from build123d import *

# Parameters (mm, degrees)
BOSS_EXTRUDE3_DEPTH = 28
FILLET1_R           = 10
SKETCH8_R           = 9.5
SKETCH8_W           = 8
SKETCH8_H           = 5
CUT_EXTRUDE4_DEPTH  = 5
SKETCH10_R          = 1.75
CUT_EXTRUDE6_DEPTH  = 10
CUT_EXTRUDE9_DEPTH  = 5
SKETCH11_W          = 178.461857567
SKETCH11_H          = 75.855450753
CUT_EXTRUDE7_DEPTH  = 56
SKETCH15_W          = 24.76037583
SKETCH15_H          = 40.698494869
CUT_EXTRUDE10_DEPTH = 39


with BuildPart() as part:
    # Sketch7 → Boss-Extrude3 (new body)
    with BuildSketch(Plane.XY):
        with BuildLine():
            Line((-29.009247715, -3.56026037), (114.990752285, -3.56026037))
            ThreePointArc((114.990752285, -3.56026037), (122.672406567, -0.574706865), (126.321710983, 6.81473963))
            Line((126.321710983, 6.81473963), (124.563663285, 6.81473963))
            ThreePointArc((124.563663285, 6.81473963), (105.365752285, 7.81473963), (124.563663285, 8.81473963))
            Line((124.563663285, 8.81473963), (126.321710983, 8.81473963))
            ThreePointArc((126.321710983, 8.81473963), (125.754505842, 11.49335817), (124.563663285, 13.958842494))
            Line((124.563663285, 13.958842494), (124.563663285, 33.43973963))
            Line((124.563663285, 33.43973963), (96.563663285, 33.43973963))
            Line((96.563663285, 33.43973963), (96.563663285, 1.43973963))
            Line((96.563663285, 1.43973963), (-10.582158714, 1.43973963))
            Line((-10.582158714, 1.43973963), (-10.582158714, 33.43973963))
            Line((-10.582158714, 33.43973963), (-38.582158714, 33.43973963))
            Line((-38.582158714, 33.43973963), (-38.582158714, 13.958842494))
            ThreePointArc((-38.582158714, 13.958842494), (-39.773001272, 11.49335817), (-40.340206412, 8.81473963))
            Line((-40.340206412, 8.81473963), (-38.582158714, 8.81473963))
            ThreePointArc((-38.582158714, 8.81473963), (-19.384247715, 7.81473963), (-38.582158714, 6.81473963))
            Line((-38.582158714, 6.81473963), (-40.340206412, 6.81473963))
            ThreePointArc((-40.340206412, 6.81473963), (-36.690901996, -0.574706865), (-29.009247715, -3.56026037))
        make_face()
    extrude(amount=BOSS_EXTRUDE3_DEPTH)

    # Fillet1
    fillet1_edges = [part.edges().sort_by_distance(p)[0] for p in [
        (-10.582158714, 1.43973963, 14),
        (96.563663285, 1.43973963, 14),
    ]]
    fillet(fillet1_edges, radius=FILLET1_R)

    # Sketch8 → Cut-Extrude4 (cut)
    with BuildSketch(Plane(origin=(0, 1.43973963, 0), x_dir=(1, 0, 0), z_dir=(0, 1, 0))):
        with Locations(Location((63.990752285, -14, 0), (0, 0, 270))):
            Circle(SKETCH8_R)
        with Locations(Location((21.990752285, -14, 0), (0, 0, 270))):
            Circle(SKETCH8_R)
        with Locations((42.990752285, -14)):
            Rectangle(SKETCH8_W, SKETCH8_H)
    extrude(amount=-CUT_EXTRUDE4_DEPTH, mode=Mode.SUBTRACT)

    # Sketch10 → Cut-Extrude6 (cut)
    with BuildSketch(Plane(origin=(0, 33.43973963, 0), x_dir=(1, 0, 0), z_dir=(0, 1, 0))):
        with Locations(Location((110.490752285, -14, 0), (0, 0, 180))):
            Circle(SKETCH10_R)
        with Locations(Location((-24.509247715, -14, 0), (0, 0, 180))):
            Circle(SKETCH10_R)
    extrude(amount=-CUT_EXTRUDE6_DEPTH, mode=Mode.SUBTRACT)

    # Sketch13 → Cut-Extrude9 (cut)
    with BuildSketch(Plane(origin=(0, 33.43973963, 0), x_dir=(1, 0, 0), z_dir=(0, 1, 0))):
        Polygon((108.61436391, -17.25), (112.36714066, -17.25), (114.243529035, -14), (112.36714066, -10.75), (108.61436391, -10.75), (106.737975536, -14), align=None)
        Polygon((-20.756470965, -14), (-22.63285934, -10.75), (-26.38563609, -10.75), (-28.262024464, -14), (-26.38563609, -17.25), (-22.63285934, -17.25), align=None)
    extrude(amount=-CUT_EXTRUDE9_DEPTH, mode=Mode.SUBTRACT)

    # Sketch11 → Cut-Extrude7 (cut)
    with BuildSketch(Plane.XY.offset(28)):
        with Locations((7.260936379, 24.571309344)):
            Rectangle(SKETCH11_W, SKETCH11_H)
    extrude(amount=-CUT_EXTRUDE7_DEPTH, mode=Mode.SUBTRACT)

    # Sketch15 → Cut-Extrude10 (cut)
    with BuildSketch(Plane.ZY.offset(-96.491865162)):
        with Locations((20.2732889, 14.243484204)):
            Rectangle(SKETCH15_W, SKETCH15_H)
    extrude(amount=-CUT_EXTRUDE10_DEPTH, mode=Mode.SUBTRACT)


solid = part.part
The listing builds one solid part. Answer for the finished solid, in the listing's coordinates (mm). A direction names the side the tool comes from. Give positions to 0.01 mm unless a question says otherwise; leave off trailing zeros. Write each loop counter-clockwise with the first axis right and the second up, starting at its lowest first coordinate (ties: lowest second). Pieces come first, ordered by that corner, then holes.
Item 1: Section C-C, the plane z = 4.75 is taken. Write down the section's boundary in (x, y) (3 decimals), plus the area to 3 significant figures.
Item 2: Find the intervals of material crossed by line 1 along X through (y, z) = (20.5, 6.5); line 2 along Y through (x, z) = (112.5, 4); line 3 along X through (y, z) = (1, 6.25), in increasing order.
Item 3: Section B-B, the plane y = 1 is taken. Write down the section's boundary in (x, z), plus the area to 3 significant figures.
Item 4: Which of the six approach directions +Z, -Z, +X, -X, +Y, -Y give full straight-line access (tool end or side, diameter ignored) to faces 4 (the flat face through (106, -3.56, 4)), 5 (the flat face through (125, 8.815, 4)), 6 (the flat face through (96.564, 23, 4))?
Item 5: Determine the mould class of faces 1 (the flat face through (124.564, 24, 4)), 2 (the flat face through (111, 33.44, 4)), 3 (the cylindrical face through (105.374, 7.406, 3.891)) for opening direction X: released by +X, released by -X, zero draft, split by the parting line, or undercut.
Item 6: Section D-D, the plane y = 29.5 is taken. Write down the section's boundary in (x, z), plus the area to 3 significant figures.
Item 7: Flat-ended cylindrical pins translate along their axes: P1, Ø1.4, axis at x = 125.5, z = 2.5, coming from the -Y side; P2, Ø1.5, axis at x = 123, z = 3, coming from the -Y side; P3, Ø2.5, axis at y = 21.5, z = 4.5, coming from the -X side. Find the tip coordinate at first contact, or state that the pin passes through.
Item 8: Section A-A, the plane x = 106 is taken. Write down the section's boundary in (y, z).
Completed:
1. outline: (96.492, -3.56) - (114.991, -3.56) arc R11.375 ccw to (126.322, 6.815) - (124.564, 6.815) arc R9.625 cw (long way) to (124.564, 8.815) - (126.322, 8.815) arc R11.375 ccw to (124.564, 13.959) - (124.564, 33.44) - (96.564, 33.44) - (96.564, 11.44) arc R10 cw to (96.492, 10.244) - close
1. area: 743 mm2
2. line 1: x = 96.56 to 124.56
2. line 2: y = -3.56 to -1.48, 17.11 to 33.44
2. line 3: x = 96.49 to 108.19, 121.79 to 124.1
3. outline: (96.49, 0) - (108.19, 0) - (108.19, 7.89) - (96.49, 7.89) - close; (121.79, 0) - (124.1, 0) - (124.1, 7.89) - (121.79, 7.89) - close
3. area: 111 mm2
4. face 4: +Z, -Z, +X, -X, -Y
4. face 5: +Z, -Z, +X
4. face 6: +Z, -Z, -X, +Y
5. face 1: released by +X
5. face 2: zero draft
5. face 3: undercut
6. outline: (96.56, 0) - (124.56, 0) - (124.56, 7.89) - (96.56, 7.89) - close
6. area: 221 mm2
7. P1: stops at y = 2.06
7. P2: stops at y = -0.94
7. P3: stops at x = 96.56
8. outline: (-3.56, 0) - (4.38, 0) - (4.38, 7.89) - (-3.56, 7.89) - close; (11.25, 0) - (33.44, 0) - (33.44, 7.89) - (11.25, 7.89) - close
